```python
from build123d import *

# Parameters (mm, degrees)
BOSS_EXTRUDE1_DEPTH = 24
SKETCH3_R           = 4
SKETCH3_R_2         = 1.5
CUT_EXTRUDE2_DEPTH  = 4
SKETCH6_R           = 4
SKETCH6_R_2         = 1.5
CUT_EXTRUDE3_DEPTH  = 4
FILLET1_R           = 5


with BuildPart() as part:
    # Sketch1 → Boss-Extrude1 (new body)
    with BuildSketch(Plane.XY):
        Polygon((-35.947712149, -38.738038278), (-35.947712149, 46.261961722), (5.197050303, 46.261961722), (5.197050303, 50.261961722), (-39.947712149, 50.261961722), (-39.947712149, -38.738038278), align=None)
    extrude(amount=BOSS_EXTRUDE1_DEPTH)

    # Sketch3 → Cut-Extrude2 (cut)
    with BuildSketch(Plane.ZY.offset(39.947712149)):
        with Locations((12, -26.738038278)):
            Circle(SKETCH3_R)
        with Locations((20, -26.738038278)):
            Circle(SKETCH3_R_2)
        with Locations((12, -34.738038278)):
            Circle(SKETCH3_R_2)
        with Locations((4, -26.738038278)):
            Circle(SKETCH3_R_2)
        with Locations((12, -18.738038278)):
            Circle(SKETCH3_R_2)
    extrude(amount=-CUT_EXTRUDE2_DEPTH, mode=Mode.SUBTRACT)

    # Sketch6 → Cut-Extrude3 (cut)
    with BuildSketch(Plane(origin=(0, 50.261961722, 0), x_dir=(1, 0, 0), z_dir=(0, 1, 0))):
        with Locations((-7.947712149, -12)):
            Circle(SKETCH6_R)
        with Locations((0.052287851, -12)):
            Circle(SKETCH6_R_2)
        with Locations((-7.947712149, -20)):
            Circle(SKETCH6_R_2)
        with Locations((-15.947712149, -12)):
            Circle(SKETCH6_R_2)
        with Locations((-7.947712149, -4)):
            Circle(SKETCH6_R_2)
    extrude(amount=-CUT_EXTRUDE3_DEPTH, mode=Mode.SUBTRACT)

    # Fillet1
    fillet1_edges = [part.edges().sort_by_distance(p)[0] for p in [
        (-35.947712149, 46.261961722, 12),
        (-39.947712149, 50.261961722, 12),
        (-37.947712149, -38.738038278, 24),
        (-37.947712149, -38.738038278, 0),
    ]]
    fillet(fillet1_edges, radius=FILLET1_R)


solid = part.part
```
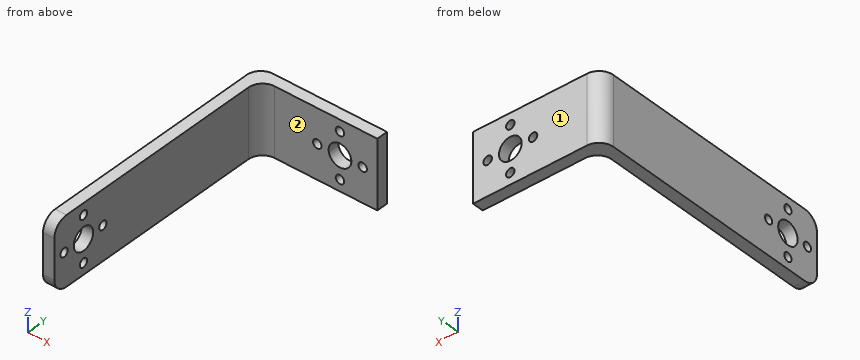
For this review, take the finished solid that the model builds, in its own axes (mm). Face numbers are marked on the shaded views. A direction names the side the tool comes from. Coordinates: 2 decimals unless noted, no trailing zeros. Loops run counter-clockwise (first coordinate to the right, second up) from the corner with the lowest first, then second, coordinate; pieces in that order, holes last.
1. Add section B-B, the plane x = -16.5. Give the boundary of the cut face in (y, z).
2. Add section C-C, the plane z = 4. Give the boundary of the cut face in (x, y).
3. Add section D-D, the plane x = -26. Give the boundary of the cut face in (y, z), then the cut area to 3 significant figures.
4. For the marked faces 1 and 2, list the 3-axis set-ups (+Z, -Z, +X, -X, +Y, -Y) from which the entire face can be reached by the end or side of a thin tool; tool diameter is ignored.
5. For line 1 (X direction, y = 47.25, z = 12); line 2 (X direction, y = 48.4, z = 12); line 3 (X direction, y = 48.5, z = 20), list the stretches that pass through material, from the lowest coordinate up.
6. Insertion check: P1, Ø6, axis at y = 4.5, z = 8.5, coming from the +X side; P2, Ø5, axis at x = -7.95, z = 20, coming from the -Y side; P3, Ø5, axis at x = 0.05, z = 12, coming from the +Y side. Each pin has a flat end and moves straight along its axis. Give the tip position at first contact, or say it passes through.
7. Add section A-A, the plane z = 12. Count the separate pieces of the cut face and the enclosed holes in it, then the cut area to 3 significant figures.
Result:
1. outline: (46.26, 0) - (50.26, 0) - (50.26, 10.61) - (46.26, 10.61) - close; (46.26, 13.39) - (50.26, 13.39) - (50.26, 24) - (46.26, 24) - close
2. outline: (-39.95, -38.64) - (-35.95, -38.64) - (-35.95, -28.24) - (-39.95, -28.24) - close; (-39.95, -25.24) - (-35.95, -25.24) - (-35.95, 41.26) arc R5 cw to (-30.95, 46.26) - (-9.45, 46.26) - (-9.45, 50.26) - (-34.95, 50.26) arc R5 ccw to (-39.95, 45.26) - close; (-6.45, 46.26) - (5.2, 46.26) - (5.2, 50.26) - (-6.45, 50.26) - close
3. outline: (46.26, 0) - (50.26, 0) - (50.26, 24) - (46.26, 24) - close
3. area: 96.0 mm2
4. face 1: +Z, -Z, +X, -X, +Y
4. face 2: +Z, -Z, +X, -Y
5. line 1: x = -39.54 to -17.45, -14.45 to -11.95, -3.95 to -1.45, 1.55 to 5.2
5. line 2: x = -38.84 to -17.45, -14.45 to -11.95, -3.95 to -1.45, 1.55 to 5.2
5. line 3: x = -38.76 to -9.45, -6.45 to 5.2
6. P1: stops at x = -35.95
6. P2: stops at y = 46.26
6. P3: stops at y = 50.26
7. separate pieces: 7
7. enclosed holes: 0
7. area: 409 mm2
